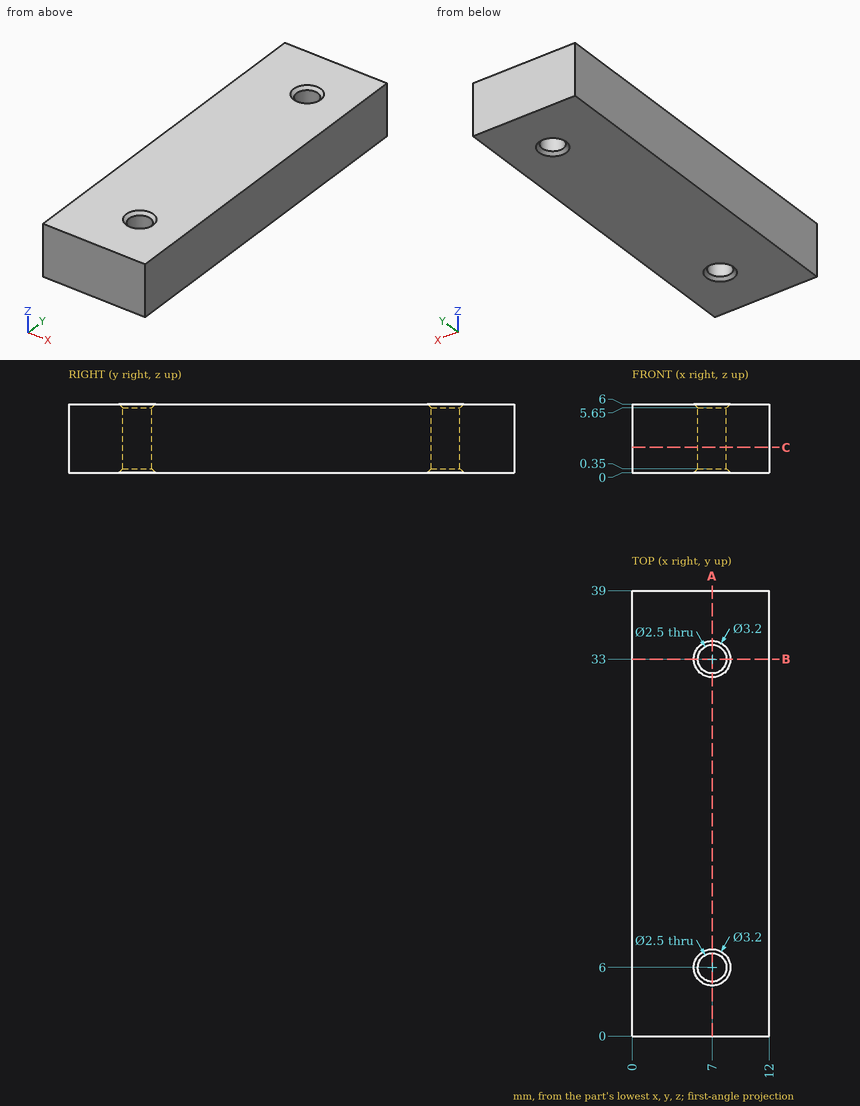
The figure shows three views and two pictorial views of one solid part (mm, origin at its lowest corner). Answer the questions. Coordinates: 2 decimals unless noted, no trailing zeros. Loops run counter-clockwise (first coordinate to the right, second up) from the corner with the lowest first, then second, coordinate; pieces in that order, holes last.
1) Find the intervals of material crossed by L1, parallel to Y at x = 7, z = 2.05; L2, parallel to Y at x = 6, z = 4.8; L3, parallel to X at y = 6, z = 2.4, in increasing order.
2) Flat-ended cylindrical pins translate along their axes: pin 1 Ø3 at (x, y) = (7, 33) entering from -Z; pin 2 Ø1.5 at (x, y) = (7, 6) entering from -Z. Find the tip coordinate at first contact, or state that the pin passes through.
3) Find section B-B on y = 33. Write down the section's boundary in (x, z).
4) Find section A-A on x = 7. Write down the section's boundary in (y, z), then the cut area to 3 significant figures.
5) Find section C-C on z = 2.2. Write down the section's boundary in (x, y).
Values:
1. L1: y = 0 to 4.75, 7.25 to 31.75, 34.25 to 39
1. L2: y = 0 to 5.25, 6.75 to 32.25, 33.75 to 39
1. L3: x = 0 to 5.75, 8.25 to 12
2. pin 1: stops at z = 0.1
2. pin 2: passes through
3. outline: (0, 0) - (5.4, 0) - (5.75, 0.35) - (5.75, 5.65) - (5.4, 6) - (0, 6) - close; (8.25, 0.35) - (8.6, 0) - (12, 0) - (12, 6) - (8.6, 6) - (8.25, 5.65) - close
4. outline: (0, 0) - (4.4, 0) - (4.75, 0.35) - (4.75, 5.65) - (4.4, 6) - (0, 6) - close; (7.25, 0.35) - (7.6, 0) - (31.4, 0) - (31.75, 0.35) - (31.75, 5.65) - (31.4, 6) - (7.6, 6) - (7.25, 5.65) - close; (34.25, 0.35) - (34.6, 0) - (39, 0) - (39, 6) - (34.6, 6) - (34.25, 5.65) - close
4. area: 204 mm2
5. outline: (0, 0) - (12, 0) - (12, 39) - (0, 39) - close; hole circle Ø2.5 at (7, 6); hole circle Ø2.5 at (7, 33)
